Print and shaded views of the part. All mm, measured from the part's lowest x, y and z. Round coordinates to 2 decimals unless told otherwise and drop trailing zeros. Order: outer loops, then holes, each group sorted by start corner. A loop starts at its lowest first (then second) coordinate and runs counter-clockwise, first axis right, second up. Notation, with made-up numbers: (79.5, 19) -> (118.5, 19) arc R13 cw to (118.5, 38) -> close; hole circle Ø8 at (-5, 63). An arc over 180 degrees is marked (long way). Answer as CSV lines item,"result". Start each with the question number.
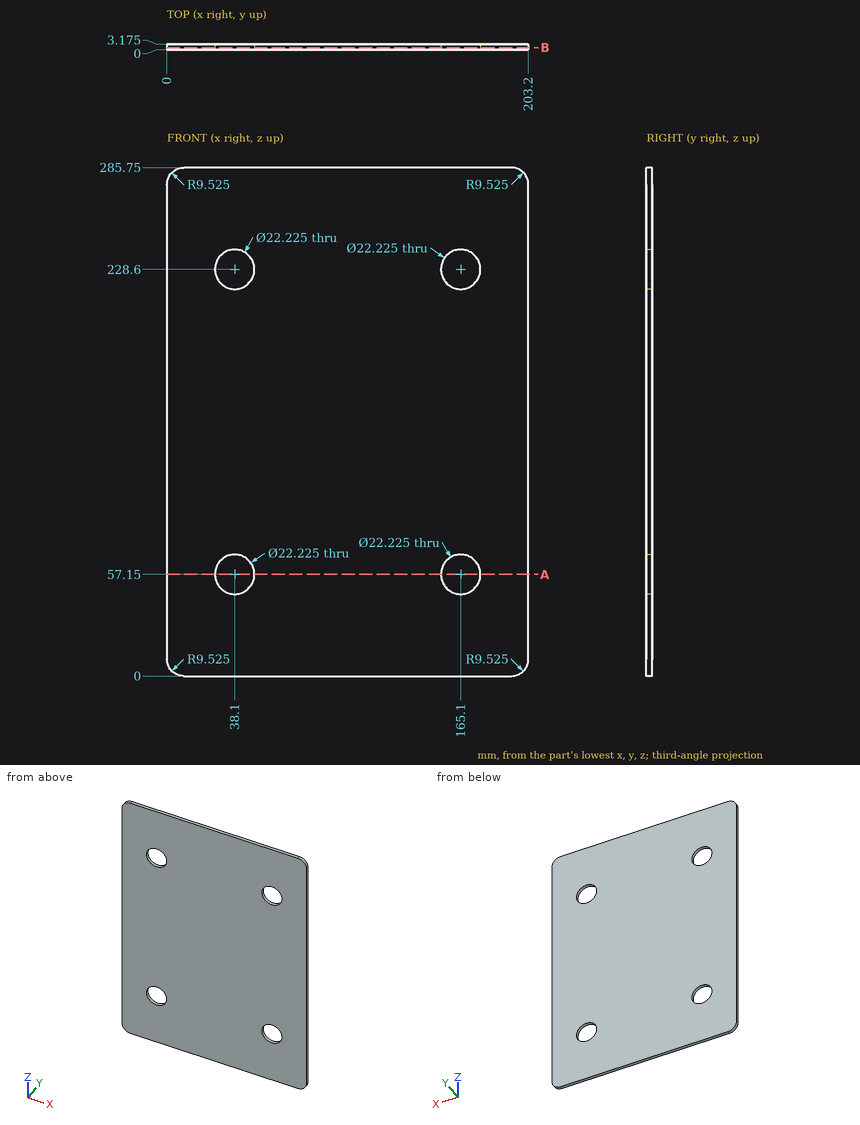
Item 1: Band-saw the part on B-B, the plane y = 1.1. Count the separate pieces of the cut face and the enclosed holes in it, and give its area (3 significant figures).
Item 2: Probe line 1 (X direction, y = 1, z = 228.6); line 2 (Z direction, x = 168.5, y = 2.85); line 3 (X direction, y = 2.7, z = 50). List the from-to ranges inside material, lowest first.
Item 3: Pin check, flat tips, straight feed: pin 1 (13.5 mm diameter, centred on x = 38.1, z = 57.15, fed in from +Y); pin 2 (1 mm diameter, centred on x = 99.5, z = 115.5, fed in from -Y). Stop position of each tip, or through.
Item 4: Band-saw the part on A-A, the plane z = 57.15. Give the cut face in (x, y) (1 decimal).
Values:
1,separate pieces,"1"
1,enclosed holes,"4"
1,area,"56,400 mm²"
2,line 1,"0 to 26.99, 49.21 to 153.99, 176.21 to 203.2"
2,line 2,"0 to 46.57, 67.73 to 218.02, 239.18 to 285.75"
2,line 3,"0 to 29.59, 46.61 to 156.59, 173.61 to 203.2"
3,pin 1,"through"
3,pin 2,"y = 0"
4,outline,"(0, 0) -> (27, 0) -> (27, 3.2) -> (0, 3.2) -> close; (49.2, 0) -> (154, 0) -> (154, 3.2) -> (49.2, 3.2) -> close; (176.2, 0) -> (203.2, 0) -> (203.2, 3.2) -> (176.2, 3.2) -> close"
